Geometry check sheet. Reference: the model listing, model coordinates, mm. Coordinates: 2 decimals unless noted, no trailing zeros. Order: outer loops, then holes, each group sorted by start corner. A loop starts at its lowest first (then second) coordinate and runs counter-clockwise, first axis right, second up. Notation, with made-up numbers: (30.5, -3.5) - (67.5, -3.5) arc R16 ccw to (67.5, 22.5) - close; hole circle Ø5 at (-0.5, 24). An arc over 180 degrees is marked (long way). Return JSON: item names as keys, results as strings. Group by question number.
Item 1: Section check C-C on y = 0.6. Enter the section's corners in (x, z), then the cut area to 3 significant figures.
Item 2: Scan lines: probe 1 along X at (y, z) = (1.05, 0); probe 2 along X at (y, z) = (1.45, 0.5); probe 3 along Z at (x, y) = (0.5, 0.2). Record each from-to range of solid material in increasing order.
Item 3: Draft check along X on faces 1 (the cylindrical face through (-9.76, 0.86, -2.17)), 2 (the flat face through (-2, 2, 2)), 3 (the cylindrical face through (4.44, 0.86, -0.35)). Enter one of: pulls with the +X half, pulls with the -X half, needs draft (parallel to the pull), parting line crosses it, or undercut.
Item 4: Gauge pin test, flat end, axial feed: pin 1 (2.5 mm diameter, centred on x = 6, z = 0, fed in from -Y). Record the tip position at first contact, or that the pin passes through.
Item 5: Section check B-B on x = 0. Enter the section's corners in (y, z).
Item 6: Section check A-A on z = 0. Enter the section's corners in (x, y).
from build123d import *

# Parameters (mm, degrees)
SKETCH1_R           = 10
SKETCH1_R_2         = 1.6
SKETCH1_R_3         = 2.25
BOSS_EXTRUDE1_DEPTH = 2
CHAMFER1_SIZE       = 0.25


with BuildPart() as part:
    # Sketch1 → Boss-Extrude1 (new body)
    with BuildSketch(Plane(origin=(0, 0, 0), x_dir=(1, 0, 0), z_dir=(0, 1, 0))):
        with Locations(Location((0, 0, 0), (0, 0, 270))):
            Circle(SKETCH1_R)
        with Locations(Location((-6, 0, 0), (0, 0, 270))):
            Circle(SKETCH1_R_2, mode=Mode.SUBTRACT)
        with Locations(Location((6, 0, 0), (0, 0, 270))):
            Circle(SKETCH1_R_2, mode=Mode.SUBTRACT)
        with Locations(Location((0, 0, 0), (0, 0, 270))):
            Circle(SKETCH1_R_3, mode=Mode.SUBTRACT)
    extrude(amount=BOSS_EXTRUDE1_DEPTH)

    # Chamfer1
    chamfer1_edges = [part.edges().sort_by_distance(p)[0] for p in [
        (0, 2, -2.25),
        (0, 2, -10),
        (-6, 2, -1.6),
        (6, 2, -1.6),
    ]]
    chamfer(chamfer1_edges, length=CHAMFER1_SIZE)


solid = part.part
Computed:
{
 "1": {"outline": "circle Ø20 at (0, 0); hole circle Ø3.2 at (-6, 0); hole circle Ø4.5 at (0, 0); hole circle Ø3.2 at (6, 0)", "area": "282 mm²"},
 "2": {"probe 1": "x = -10 to -7.6, -4.4 to -2.25, 2.25 to 4.4, 7.6 to 10", "probe 2": "x = -9.99 to -7.52, -4.48 to -2.19, 2.19 to 4.48, 7.52 to 9.99", "probe 3": "z = -9.99 to -2.19, 2.19 to 9.99"},
 "3": {"face 1": "parting line crosses it", "face 2": "needs draft", "face 3": "undercut"},
 "4": {"pin 1": "passes through"},
 "5": {"outline": "(0, -10) - (1.75, -10) - (2, -9.75) - (2, -2.5) - (1.75, -2.25) - (0, -2.25) - close; (0, 2.25) - (1.75, 2.25) - (2, 2.5) - (2, 9.75) - (1.75, 10) - (0, 10) - close"},
 "6": {"outline": "(-10, 0) - (-7.6, 0) - (-7.6, 1.75) - (-7.85, 2) - (-9.75, 2) - (-10, 1.75) - close; (-4.4, 0) - (-2.25, 0) - (-2.25, 1.75) - (-2.5, 2) - (-4.15, 2) - (-4.4, 1.75) - close; (2.25, 0) - (4.4, 0) - (4.4, 1.75) - (4.15, 2) - (2.5, 2) - (2.25, 1.75) - close; (7.6, 0) - (10, 0) - (10, 1.75) - (9.75, 2) - (7.85, 2) - (7.6, 1.75) - close"}
}
